Verification items for the finished model (mm, model axes). A direction names the side the tool comes from. Give positions to 0.01 mm unless a question says otherwise; leave off trailing zeros. Write each loop counter-clockwise with the first axis right and the second up, starting at its lowest first coordinate (ties: lowest second). Pieces come first, ordered by that corner, then holes. Notation, with made-up numbers: M 12,13.25 L 38,13.25 A19 ccw 38,38.25 Z; hole C -2.75,-17.75 d6. An arc over 180 degrees is marked long. Answer as a JSON object with one key per item and string values.
```python
from build123d import *

# Parameters (mm, degrees)
BOSS_EXTRUDE1_DEPTH = 95.25
BOSS_EXTRUDE2_DEPTH = 3
BOSS_EXTRUDE3_DEPTH = 95.25


with BuildPart() as part:
    # Sketch1 → Boss-Extrude1 (new body)
    with BuildSketch(Plane.XY):
        with BuildLine():
            Line((241, 0), (3, 0))
            ThreePointArc((3, 0), (0.493692681, 28.205363915), (9.651836979, 55))
            Line((9.651836979, 55), (183.85, 147))
            Line((183.85, 147), (185.251015228, 144.347236096))
            Line((185.251015228, 144.347236096), (14.182291728, 54))
            ThreePointArc((14.182291728, 54), (4.732417832, 29.325080272), (7, 3))
            Line((7, 3), (241, 3))
            Line((241, 3), (241, 0))
        make_face()
    extrude(amount=BOSS_EXTRUDE1_DEPTH)

    # Sketch2 → Boss-Extrude2 (add)
    with BuildSketch(Plane(origin=(0, 0, 0), x_dir=(-1, 0, 0), z_dir=(0, 0, -1))):
        with BuildLine():
            Line((-53.8, 78.316152866), (-53.8, 0))
            Line((-53.8, 0), (-3, 0))
            ThreePointArc((-3, 0), (-0.493692681, 28.205363915), (-9.651836979, 55))
            Line((-9.651836979, 55), (-53.8, 78.316152866))
        make_face()
    extrude(amount=-BOSS_EXTRUDE2_DEPTH)

    # Sketch3 → Boss-Extrude3 (add)
    with BuildSketch(Plane(origin=(0, 0, 0), x_dir=(-1, 0, 0), z_dir=(0, 0, -1))):
        Polygon((-9.651836979, 55), (-2.507196918, 73.680313659), (-5.309243966, 74.752009668), (-12.324009257, 56.411265454), align=None)
    extrude(amount=-BOSS_EXTRUDE3_DEPTH)


solid = part.part
```
1) Access from +Z, -Z, +X, -X, +Y, -Y to the whole of each face (thin tool, end or side, straight path). Record for faces 4 (the face through (8.768, 65.71, 46.958)), 5 (the face through (4.786, 29.694, 48.479)), 6 (the face through (6.13, 64.21, 46.96)).
Completed:
{"face 4": "+Z, -Z, +Y", "face 5": "+Z, +X", "face 6": "+Z, -Z, -X"}
2) Go/stop test with flat-tipped pins: pin 1 (8 mm diameter, centred on y = 101.5, z = 24.5, fed in from -X); pin 2 (10 mm diameter, centred on y = 114, z = 30.5, fed in from -X); pin 3 (1.5 mm diameter, centred on y = 22, z = 1.5, fed in from +X). Record where each tip stops, or that it passes through.
Completed:
{"pin 1": "stops at x = 90.12", "pin 2": "stops at x = 111.9", "pin 3": "stops at x = 53.8"}
3) Section check D-D on x = 17. Record the boundary of the cut face in (y, z).
Completed:
{"outline": "M 0,0 L 58.88,0 L 58.88,95.25 L 55.49,95.25 L 55.49,3 L 3,3 L 3,95.25 L 0,95.25 Z"}
4) Section check B-B on y = 61.5. Record the boundary of the cut face in (x, z).
Completed:
{"outline": "M 7.17,0 L 10.38,0 L 10.38,95.25 L 7.17,95.25 Z; M 21.96,0 L 53.8,0 L 53.8,3 L 28.38,3 L 28.38,95.25 L 21.96,95.25 Z"}
5) Section check C-C on x = 171.5. Record the boundary of the cut face in (y, z).
Completed:
{"outline": "M 0,0 L 3,0 L 3,95.25 L 0,95.25 Z; M 137.08,0 L 140.48,0 L 140.48,95.25 L 137.08,95.25 Z"}
6) Release check for a two-part mould opening along Y. For faces 1 (the face through (29, 31, 3)), 2 (the face through (96.886, 101.072, 46.958)), 3 (the face through (68, 85, 95.25)) record: pulls with the +Y half, pulls with the -Y half, needs draft (parallel to the pull), parting line crosses it, or undercut.
Completed:
{"face 1": "undercut", "face 2": "pulls with the +Y half", "face 3": "needs draft"}
7) Section check A-A on z = 19. Record the boundary of the cut face in (x, y), and give its area (3 significant figures).
Completed:
{"outline": "M 2.51,73.68 L 9.65,55 A68.24 ccw 3,0 L 241,0 L 241,3 L 7,3 A59 cw 14.18,54 L 185.25,144.35 L 183.85,147 L 12.32,56.41 L 5.31,74.75 Z", "area": "1,590 mm2"}
8) Thickness scan on L1, parallel to Y at x = 226, z = 43.5; L2, parallel to Y at x = 21, z = 86.5; L3, parallel to Y at x = 90, z = 25.5. Record the ranges inside material, lowest first.
Completed:
{"L1": "y = 0 to 3", "L2": "y = 0 to 3, 57.6 to 60.99", "L3": "y = 0 to 3, 94.04 to 97.43"}
